```python
from build123d import *

# Parameters (mm, degrees)
F0_R     = 5
F1_DEPTH = 6
F2_R     = 0.4


with BuildPart() as f1:
    # F0 (on Right) → F1 (new body)
    with BuildSketch(Plane.YZ):
        Polygon((4.469955, 7.742188), (-4.469955, 7.742188), (-8.939909, 0), (-4.469955, -7.742188), (4.469955, -7.742188), (8.939909, 0), align=None)
        Circle(F0_R, mode=Mode.SUBTRACT)
    extrude(amount=-F1_DEPTH)

    # F2
    f2_edges = [f1.edges().sort_by_distance(p)[0] for p in [
        (-3, 4.469955, 7.742188),
        (-3, 8.939909, 0),
        (-3, 4.469955, -7.742188),
        (-3, -4.469955, -7.742188),
        (-3, -8.939909, 0),
        (0, -6.704932, -3.871094),
        (0, 0, -7.742188),
        (0, 6.704932, -3.871094),
        (0, 6.704932, 3.871094),
        (-6, 6.704932, 3.871094),
        (-6, 6.704932, -3.871094),
        (-6, 0, -7.742188),
        (-6, -6.704932, -3.871094),
        (-3, -4.469955, 7.742188),
        (0, -6.704932, 3.871094),
        (-6, -6.704932, 3.871094),
        (0, 0, 7.742188),
        (-6, 0, 7.742188),
    ]]
    fillet(f2_edges, radius=F2_R)


solid = f1.part
```
For this review, take the finished solid that the model builds, in its own axes (mm). Coordinates: 2 decimals unless noted, no trailing zeros. Order: outer loops, then holes, each group sorted by start corner. A loop starts at its lowest first (then second) coordinate and runs counter-clockwise, first axis right, second up. Notation, with made-up numbers: (-32.5, 80.5) - (26.5, 80.5) arc R11 ccw to (26.5, 86.5) - close; hole circle Ø2 at (88, -22.5). An arc over 180 degrees is marked (long way). Answer as a JSON object with one key per item and string values. Group by question number.
1. The part is to be moulded in two halves that separate along Z. For faces 1 (the flat face through (-3, 0, -7.742)), 2 (the cylindrical face through (-2.96, -1.08, -4.88)), 3 (the flat face through (0, 2, 5)), say which applies: pulls with the +Z half, pulls with the -Z half, needs draft (parallel to the pull), parting line crosses it, or undercut.
2. We need section A-A on y = -3. State the section outline as (x, z) points.
3. We need section B-B on x = -2.5. State the section outline as (y, z) points.
4. For probe 1 along Z at (x, y) = (-2.55, 0); probe 2 along Z at (x, y) = (-2.5, 2); probe 3 along Y at (x, z) = (-0.25, 1.75), list the stretches that pass through material, from the lowest coordinate up.
5. Clearance check with flat-ended pins moving along their axes: P1, Ø6, axis at y = 0, z = 0, coming from the -X side; P2, Ø2, axis at x = -2.5, y = -5.5, coming from the -Z side; P3, Ø2, axis at x = -3, z = 3.5, coming from the -Y side. State where each tip first meets the part, or that it passes through.
6. We need section C-C on y = 0. State the section outline as (x, z) points, then the cut area to 3 significant figures.
Final values:
{
 "1": {"face 1": "pulls with the -Z half", "face 2": "undercut", "face 3": "needs draft"},
 "2": {"outline": "(-6, -7.34) arc R0.4 ccw to (-5.6, -7.74) - (-0.4, -7.74) arc R0.4 ccw to (0, -7.34) - (0, -4) - (-6, -4) - close; (-6, 4) - (0, 4) - (0, 7.34) arc R0.4 ccw to (-0.4, 7.74) - (-5.6, 7.74) arc R0.4 ccw to (-6, 7.34) - close"},
 "3": {"outline": "(-8.82, -0.2) - (-4.59, -7.54) arc R0.4 ccw to (-4.24, -7.74) - (4.24, -7.74) arc R0.4 ccw to (4.59, -7.54) - (8.82, -0.2) arc R0.4 ccw to (8.82, 0.2) - (4.59, 7.54) arc R0.4 ccw to (4.24, 7.74) - (-4.24, 7.74) arc R0.4 ccw to (-4.59, 7.54) - (-8.82, 0.2) arc R0.4 ccw to start; hole circle Ø10 at (0, 0)"},
 "4": {"probe 1": "-7.74 to -5, 5 to 7.74", "probe 2": "-7.74 to -4.58, 4.58 to 7.74", "probe 3": "-7.9 to -4.68, 4.68 to 7.9"},
 "5": {"P1": "through", "P2": "z = -7.65", "P3": "y = -7.5"},
 "6": {"outline": "(-6, -7.34) arc R0.4 ccw to (-5.6, -7.74) - (-0.4, -7.74) arc R0.4 ccw to (0, -7.34) - (0, -5) - (-6, -5) - close; (-6, 5) - (0, 5) - (0, 7.34) arc R0.4 ccw to (-0.4, 7.74) - (-5.6, 7.74) arc R0.4 ccw to (-6, 7.34) - close", "area": "32.8 mm²"}
}
